Autodesk Inventor part; units mm, degrees
ref_plane "YZ Plane" through (0, 0, 0) normal (1, 0, 0) x (0, 1, 0)
ref_plane "XZ Plane" through (0, 0, 0) normal (0, 1, 0) x (-1, 0, 0)
ref_plane "XY Plane" through (0, 0, 0) normal (0, 0, 1) x (1, 0, 0)
sketch "Sketch1" plane through (0, 0, 0) normal (0, 0, 1) x (1, 0, 0)
  circle A0 centre (0, 0) radius 10
  circle A1 centre (0, 0) radius 20
  line L0 (-15, 0) -> (15, 0)
  line L1 (15, 0) -> (15, 50)
  line L2 (15, 50) -> (-15, 50)
  line L3 (-15, 50) -> (-15, 0)
  point P0 (-15, 13.2288)
  point P1 (15, 13.2288)
  dimension "d0" = 20
  dimension "d1" = 40
  dimension "d2" = 30
  dimension "d3" = 50
extrude "Extrusion1" add sketch "Sketch1" along normal blind 20
sketch "Sketch2" plane through (0, 0, 20) normal (0, 0, 1) x (1, 0, 0)
  circle A0 centre (0, 0) radius 10
  dimension "d6" = 20
extrude "Extrusion2" cut sketch "Sketch2" against normal blind 15
sketch "Sketch4" plane through (-15, 13.2288, 0) normal (-1, 0, 0) x (0, 0, 1)
  line L0 (0, 36.7712) -> (20, 36.7712)
  line L1 (0, 0) -> (0, 36.7712)
  line L2 (20, 36.7712) -> (0, 36.7712)
  line L3 (0, 36.7712) -> (0, 0)
  line L4 (0, 0) -> (20, 0)
  line L5 (20, 0) -> (20, 36.7712)
  line L6 (0, 0) -> (20, 0)
  line L7 (20, 36.7712) -> (10, 36.7712)
  line L8 (10, 36.7712) -> (10, 0)
  line L9 (10, 0) -> (20, 0)
  line L10 (20, 0) -> (20, 36.7712)
  line L11 (10, 0) -> (16, 0)
  line L12 (16, 0) -> (16, 25)
  line L13 (16, 25) -> (10, 25)
  line L14 (10, 25) -> (10, 0)
  line L15 (10, 25) -> (4, 25)
  line L16 (4, 25) -> (4, 0)
  line L17 (4, 0) -> (10, 0)
  line L18 (10, 0) -> (10, 25)
  line L19 (4, 25) -> (16, 25)
  line L20 (16, 25) -> (16, 30.0005)
  line L21 (16, 30.0005) -> (4, 30.0005)
  line L22 (4, 30.0005) -> (4, 25)
  line L23 (4, 30.0005) -> (16, 30.0005)
  line L24 (16, 30.0005) -> (16, 7.0005)
  line L25 (16, 7.0005) -> (4, 7.0005)
  line L26 (4, 7.0005) -> (4, 30.0005)
  line L27 (10, 7.0005) -> (16, 7.0005)
  line L28 (16, 7.0005) -> (16, 0)
  line L29 (16, 0) -> (10, 0)
  line L30 (10, 0) -> (10, 7.0005)
  point P0 (0, -13.2288)
  dimension "d13" = 6
  dimension "d14" = 25
  dimension "d15" = 6
  dimension "d16" = 23
extrude "Extrusion3" cut sketch "Sketch4" against normal blind 23 contours L21 L20 L13 L8 | L8 L15 L22 L21 | L13 L12 L25 L8 | L8 L25 L16 L15
sketch "Sketch6" plane through (-15, 13.2288, 0) normal (-1, 0, 0) x (0, 0, 1)
  line L0 (4, 7.0005) -> (4, 30.0005)
  line L1 (4, 7.0005) -> (16, 7.0005)
  line L2 (16, 7.0005) -> (16, 2.2005)
  line L3 (16, 2.2005) -> (4, 2.2005)
  line L4 (4, 2.2005) -> (4, 7.0005)
  line L5 (4, 30.0005) -> (16, 30.0005)
  line L6 (16, 30.0005) -> (16, 34.8005)
  line L7 (16, 34.8005) -> (4, 34.8005)
  line L8 (4, 34.8005) -> (4, 30.0005)
  point P0 (0, -13.2288)
  dimension "d19" = 12
  dimension "d20" = 4.8
  dimension "d21" = 4.8
extrude "Extrusion4" cut sketch "Sketch6" against normal blind 16
sketch "Sketch7" plane through (1, 13.2288, 0) normal (-1, 0, 0) x (0, 0, 1)
  line L0 (4, 30.0005) -> (16, 30.0005)
  line L1 (4, 30.0005) -> (10, 30.0005)
  line L2 (10, 30.0005) -> (10, 32.5005)
  line L3 (10, 32.5005) -> (4, 32.5005)
  line L4 (4, 32.5005) -> (4, 30.0005)
  circle A0 centre (10, 32.5005) radius 0.75
  line L5 (16, 7.0005) -> (4, 7.0005)
  line L6 (16, 7.0005) -> (16, 2.2005)
  line L7 (4, 7.0005) -> (16, 7.0005)
  line L8 (16, 7.0005) -> (16, 4.5005)
  line L9 (16, 4.5005) -> (4, 4.5005)
  line L10 (4, 4.5005) -> (4, 7.0005)
  line L11 (10, 4.5005) -> (4, 4.5005)
  line L12 (4, 4.5005) -> (4, 7.0005)
  line L13 (4, 7.0005) -> (10, 7.0005)
  line L14 (10, 7.0005) -> (10, 4.5005)
  circle A1 centre (10, 4.5005) radius 0.75
  point P0 (0, -13.2288)
  dimension "d24" = 2.5
  dimension "d25" = 1.5
  dimension "d26" = 2.5
  dimension "d27" = 1.5
extrude "Extrusion5" cut sketch "Sketch7" against normal blind 8 contours A0 L3 L2 | L2 L3 A0 | A1 L9 L14 | L14 L9 A1 | A1 L9
sketch "Sketch8" plane through (15, 13.2288, 0) normal (1, 0, 0) x (0, 0, -1)
  line L0 (0, 36.7712) -> (0, 0)
  line L1 (-20, 36.7712) -> (-20, 0)
  line L2 (0, 36.7712) -> (-20, 36.7712)
  line L3 (-20, 36.7712) -> (-20, 26.7712)
  line L4 (-20, 26.7712) -> (0, 26.7712)
  line L5 (0, 26.7712) -> (0, 36.7712)
  line L6 (0, 26.7712) -> (-20, 26.7712)
  line L7 (-20, 26.7712) -> (-20, 18.7712)
  line L8 (-20, 18.7712) -> (0, 18.7712)
  line L9 (0, 18.7712) -> (0, 26.7712)
  line L10 (0, 26.7712) -> (-10, 26.7712)
  line L11 (-10, 26.7712) -> (-10, 18.7712)
  line L12 (-10, 18.7712) -> (0, 18.7712)
  line L13 (0, 18.7712) -> (0, 26.7712)
  line L14 (-10, 26.7712) -> (-5, 26.7712)
  line L15 (-5, 26.7712) -> (-5, 22.7712)
  line L16 (-5, 22.7712) -> (-10, 22.7712)
  line L17 (-10, 22.7712) -> (-10, 26.7712)
  line L18 (-10, 22.7712) -> (-15, 22.7712)
  line L19 (-15, 22.7712) -> (-15, 26.7712)
  line L20 (-15, 26.7712) -> (-10, 26.7712)
  line L21 (-10, 26.7712) -> (-10, 22.7712)
  point P0 (0, -13.2288)
  dimension "d30" = 10
  dimension "d31" = 8
  dimension "d32" = 5
  dimension "d33" = 5
extrude "Extrusion6" cut sketch "Sketch8" against normal blind 15.8125 contours L15 L16 L11 L4 | L11 L18 L19 L4
sketch "Sketch9" plane through (0, 0, 5) normal (0, 0, 1) x (1, 0, 0)
  circle A0 centre (0, 0) radius 1
  circle A1 centre (7, 0) radius 1.5
  circle A2 centre (0, 0) radius 1.5
  circle A3 centre (-7, 0) radius 1.5
  dimension "d36" = 2
  dimension "d37" = 3
  dimension "d38" = 3
  dimension "d39" = 3
extrude "Extrusion7" cut sketch "Sketch9" against normal blind 8 contours A0 | A1 | A2 | A3
sketch "Sketch10" plane through (-15, 50, 0) normal (0, 1, 0) x (1, 0, 0)
  line L0 (0, 0) -> (0, -20)
  line L1 (0, 0) -> (29.4792, 0)
  line L2 (29.4792, 0) -> (29.4792, -20)
  line L3 (29.4792, -20) -> (0, -20)
  line L4 (0, -20) -> (0, 0)
  point P0 (15, 0)
extrude "Extrusion8" add sketch "Sketch10" along normal blind 10
sketch "Sketch11" plane through (0, 0, 0) normal (0, 0, -1) x (-1, 0, 0)
  line L0 (15, 13.2288) -> (15, 60)
  line L1 (-15, 13.2288) -> (-15, 50)
  line L2 (15, 60) -> (-15, 60)
  line L3 (-15, 60) -> (-15, 45)
  line L4 (-15, 45) -> (15, 45)
  line L5 (15, 45) -> (15, 60)
  line L6 (15, 45) -> (-15, 45)
  line L7 (-15, 45) -> (-15, 35)
  line L8 (-15, 35) -> (15, 35)
  line L9 (15, 35) -> (15, 45)
  point P0 (0, 0)
  dimension "d47" = 15
  dimension "d48" = 10
sketch "Sketch12" plane through (14.4792, 50, 20) normal (1, 0, 0) x (0, 0, -1)
  line L0 (20, 0) -> (20, 10)
  line L1 (0, 0) -> (20, 0)
  line L2 (20, 0) -> (20, 10)
  line L3 (20, 10) -> (0, 10)
  line L4 (0, 10) -> (0, 0)
  point P0 (20, -50)
extrude "Extrusion9" cut sketch "Sketch12" against normal blind 59.6125
sketch "Sketch13" plane through (-15, 50, 0) normal (0, 1, 0) x (1, 0, 0)
  line L0 (30, 0) -> (30, -20)
  line L1 (0, 0) -> (30, 0)
  line L2 (30, 0) -> (30, -20)
  line L3 (30, -20) -> (0, -20)
  line L4 (0, -20) -> (0, 0)
  point P0 (15, 0)
extrude "Extrusion10" add sketch "Sketch13" along normal blind 10
extrude "Extrusion11" add sketch "Sketch11" along normal blind 10
sketch "Sketch15" plane through (0, 0, 20) normal (0, 0, 1) x (1, 0, 0)
  line L0 (-15, 60) -> (15, 60)
  line L1 (-15, 60) -> (0, 60)
  line L2 (0, 60) -> (0, 35)
  line L3 (0, 35) -> (-15, 35)
  line L4 (-15, 35) -> (-15, 60)
  point P0 (0, 0)
  dimension "d56" = 25
extrude "Extrusion12" add sketch "Sketch15" along normal blind 10
sketch "Sketch16" plane through (0, 0, -10) normal (0, 0, -1) x (-1, 0, 0)
  line L0 (-15, 13.2288) -> (-15, 60)
  line L1 (0, 35) -> (15, 35)
  line L2 (-15, 60) -> (0, 60)
  line L3 (0, 60) -> (0, 35)
  line L4 (0, 35) -> (-15, 35)
  line L5 (-15, 35) -> (-15, 60)
  point P0 (0, 0)
extrude "Extrusion13" cut sketch "Sketch16" against normal blind 10
sketch "Sketch17" plane through (-15, 13.2288, 0) normal (-1, 0, 0) x (0, 0, 1)
  line L0 (0, 0) -> (0, 46.7712)
  line L1 (0, 46.7712) -> (10, 46.7712)
  line L2 (10, 46.7712) -> (10, 23.4712)
  line L3 (10, 23.4712) -> (0, 23.4712)
  line L4 (0, 23.4712) -> (0, 46.7712)
  circle A0 centre (10, 23.4712) radius 10
  line L5 (20, 46.7712) -> (30, 46.7712)
  line L6 (20, 0) -> (20, 46.7712)
  line L7 (30, 46.7712) -> (20, 46.7712)
  line L8 (20, 46.7712) -> (20, 36.7712)
  line L9 (20, 36.7712) -> (30, 36.7712)
  line L10 (30, 36.7712) -> (30, 46.7712)
  line L11 (30, 46.7712) -> (24, 46.7712)
  line L12 (24, 46.7712) -> (24, 36.7712)
  line L13 (24, 36.7712) -> (30, 36.7712)
  line L14 (30, 36.7712) -> (30, 46.7712)
  circle A1 centre (24, 36.7712) radius 2
  line L15 (30, 46.7712) -> (-10, 46.7712)
  line L16 (-10, 46.7712) -> (-4, 46.7712)
  line L17 (-4, 46.7712) -> (-4, 36.7712)
  line L18 (-4, 36.7712) -> (-10, 36.7712)
  line L19 (-10, 36.7712) -> (-10, 46.7712)
  circle A2 centre (-4, 36.7712) radius 2
  point P0 (0, -13.2288)
  dimension "d61" = 23.3
  dimension "d62" = 20
  dimension "d63" = 10
  dimension "d64" = 6
  dimension "d65" = 4
  dimension "d66" = 6
  dimension "d67" = 4
extrude "Extrusion14" add sketch "Sketch17" along normal blind 8 contours A2 L18 L17 | L17 L18 A2 | A1 L12 L9 | L9 A1 | L12 A1 L9
sketch "Sketch18" plane through (0, 0, 20) normal (0, 0, 1) x (1, 0, 0)
  circle A0 centre (0, 0) radius 10
extrude "Extrusion15" add sketch "Sketch18" against normal blind 16
sketch "Sketch19" plane through (0, 0, 0) normal (0, 0, -1) x (-1, 0, 0)
  circle A0 centre (0, 0) radius 1.5
  circle A1 centre (0, 0) radius 10
  dimension "d72" = 20
extrude "Extrusion16" cut sketch "Sketch19" against normal blind 16
sketch "Sketch20" plane through (0, 0, 4) normal (0, 0, -1) x (-1, 0, 0)
  circle A0 centre (0, 0) radius 1.5
  circle A1 centre (0, 0) radius 1.5
extrude "Extrusion17" cut sketch "Sketch20" against normal blind 30.0375
sketch "Sketch21" plane through (0, 0, 16) normal (0, 0, -1) x (-1, 0, 0)
  circle A0 centre (5, 0) radius 1
  circle A1 centre (-5, 0) radius 1
  point P0 (0, 0)
  dimension "d77" = 2
  dimension "d78" = 2
extrude "Extrusion18" cut sketch "Sketch21" against normal blind 138.2375
chamfer "Chamfer2" distance 8 angle 45 1 edges at (10, 0, 0)
properties part number "EndConnector"
Could you check a few things on this model? Use its own coordinates, in mm. A direction names the side the tool comes from. Round coordinates to 2 decimals unless told otherwise and drop trailing zeros. Loops run counter-clockwise (first coordinate to the right, second up) from the corner with the lowest first, then second, coordinate; pieces in that order, holes last.
Q1. I want a section at B-B (z = 18). Write out the boundary of the cut face in (x, y).
Q2. I want a section at A-A (y = 0). Write out the boundary of the cut face in (x, z).
Q3. I want a section at D-D (x = -5). Give the number of separate pieces and of enclosed holes in the cut face, and give its area (3 significant figures).
Q4. For P1, Ø16, axis at y = 37.5, z = 6.5, coming from the +X side; P2, Ø9.5, axis at y = 32.5, z = 9.5, coming from the -X side; P3, Ø3, axis at x = -4.5, z = 9.5, coming from the -Y side; P4, Ø1.6, axis at x = -5, y = 0, coming from the +Z side, each with a flat end and sliding along its axis, tell me the tip position at first contact or that it passes through.
Q5. Thinking about a two-plate mould opening in Z: for faces 4 (the flat face through (-7, 15.429, 10)), 5 (the flat face through (-2, 0, 16)), 6 (the flat face through (0, 48, 25)), which applies, pulls with the +Z half, pulls with the -Z half, needs draft (parallel to the pull), parting line crosses it, or undercut?
Q6. Please list where these lines run through material, in increasing order: L1, parallel to Z at x = 0.5, y = 40.5; L2, parallel to Z at x = -12, y = 45; L3, parallel to Y at x = 4, z = 6.
Q7. On a 3-axis mill with a long thin cutter (end or side, diameter ignored), from which of +Z, -Z, +X, -X, +Y, -Y can I reach the whole of each face in a straight line? I mean faces 1 (the flat face through (12, 38, 5)), 2 (the flat face through (-4, 32, 4)), 3 (the flat face through (-7, 35, 25)). Say none if no direction works.
Q8. I want a section at C-C (z = 24). Write out the boundary of the cut face in (x, y).
Answer below:
1. outline: (-15, 13.23) arc R20 ccw (long way) to (15, 13.23) - (15, 60) - (-15, 60) - close; hole circle Ø2 at (-5, 0); hole circle Ø3 at (0, 0); hole circle Ø2 at (5, 0)
2. outline: (-20, 0) - (-18, 0) - (-10, 8) - (-10, 16) - (-6, 16) - (-6, 20) - (-20, 20) - close; (-4, 16) - (-1.5, 16) - (-1.5, 20) - (-4, 20) - close; (1.5, 16) - (4, 16) - (4, 20) - (1.5, 20) - close; (6, 16) - (10, 16) - (10, 8) - (18, 0) - (20, 0) - (20, 20) - (6, 20) - close
3. separate pieces: 2
3. enclosed holes: 1
3. area: 1,340 mm2
4. P1: stops at x = 15
4. P2: stops at x = 8
4. P3: stops at y = -19.77
4. P4: passes through
5. face 4: undercut
5. face 5: pulls with the -Z half
5. face 6: needs draft
6. L1: z = 0 to 4, 16 to 20
6. L2: z = -10 to 4, 16 to 30
6. L3: y = -19.6 to -11.31, 11.31 to 20.23, 43.23 to 60
7. face 1: +X, -X
7. face 2: -X
7. face 3: +Z, +X, -X, -Y
8. outline: (-23, 48) - (-15, 48) - (-15, 35) - (0, 35) - (0, 60) - (-15, 60) - (-15, 52) - (-23, 52) - close
